Could you check a few things on this model? Use its own coordinates, in mm. Face numbers are marked on the shaded views. A direction names the side the tool comes from. Round coordinates to 2 decimals unless told otherwise and drop trailing zeros. Loops run counter-clockwise (first coordinate to the right, second up) from the corner with the lowest first, then second, coordinate; pieces in that order, holes last. Notation, with made-up numbers: M -31,54 L 23,54 A20 ccw 23,89 Z; hole C -33.75,9 d7. An arc over 180 degrees is marked long. Answer in a Markdown table with one row per item.
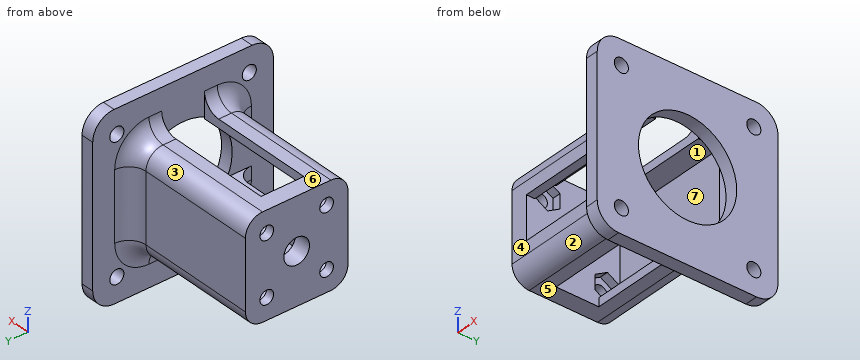
```python
from build123d import *

# Parameters (mm, degrees)
F0_W     = 24
F0_H     = 24
F0_R     = 1.6
F0_R_2   = 3
F1_DEPTH = 4
F4_DEPTH = 2
F5_DEPTH = 28
F6_W     = 42.3
F6_H     = 42.3
F6_R     = 1.65
F6_R_2   = 11.5
F7_DEPTH = 3
F8_R     = 5
F9_F1_R  = 4
F9_F2_R  = 4


with BuildPart() as f1:
    # F0 (on Right) → F1 (new body)
    with BuildSketch(Plane.YZ):
        Rectangle(F0_W, F0_H)
        with Locations((-7, -7)):
            Circle(F0_R, mode=Mode.SUBTRACT)
        with Locations((7, -7)):
            Circle(F0_R, mode=Mode.SUBTRACT)
        with Locations((-7, 7)):
            Circle(F0_R, mode=Mode.SUBTRACT)
        Circle(F0_R_2, mode=Mode.SUBTRACT)
        with Locations((7, 7)):
            Circle(F0_R, mode=Mode.SUBTRACT)
    extrude(amount=F1_DEPTH)

    # F2 (on face) → F4 (cut)
    with BuildSketch(Plane.YZ.offset(4)):
        Polygon((7, -3.6513684387), (4.1, -5.3256842194), (4.1, -8.6743157806), (7, -10.3486315613), (9.9, -8.6743157806), (9.9, -5.3256842194), align=None)
        Polygon((4.1, 5.3256842194), (7, 3.6513684387), (9.9, 5.3256842194), (9.9, 8.6743157806), (7, 10.3486315613), (4.1, 8.6743157806), align=None)
        Polygon((-9.9, 5.3256842194), (-7, 3.6513684387), (-4.1, 5.3256842194), (-4.1, 8.6743157806), (-7, 10.3486315613), (-9.9, 8.6743157806), align=None)
        Polygon((-4.1, -5.3256842194), (-7, -3.6513684387), (-9.9, -5.3256842194), (-9.9, -8.6743157806), (-7, -10.3486315613), (-4.1, -8.6743157806), align=None)
    extrude(amount=-F4_DEPTH, mode=Mode.SUBTRACT)

    # F3 (on face) → F5 (join)
    with BuildSketch(Plane.YZ.offset(4)):
        Polygon((-5, 12), (-12, 12), (-12, 5), (-10, 5), (-10, 10), (-5, 10), align=None)
        Polygon((12, 12), (5, 12), (5, 10), (10, 10), (10, -10), (5, -10), (5, -12), (12, -12), align=None)
        Polygon((-10, -5), (-12, -5), (-12, -12), (-5, -12), (-5, -10), (-10, -10), align=None)
    extrude(amount=F5_DEPTH)

    # F6 (on face) → F7 (join)
    with BuildSketch(Plane.YZ.offset(32)):
        Rectangle(F6_W, F6_H)
        with Locations((-15.5, -15.5)):
            Circle(F6_R, mode=Mode.SUBTRACT)
        with Locations((15.5, -15.5)):
            Circle(F6_R, mode=Mode.SUBTRACT)
        with Locations((-15.5, 15.5)):
            Circle(F6_R, mode=Mode.SUBTRACT)
        Circle(F6_R_2, mode=Mode.SUBTRACT)
        with Locations((15.5, 15.5)):
            Circle(F6_R, mode=Mode.SUBTRACT)
    extrude(amount=F7_DEPTH)

    # F8
    f8_edges = [f1.edges().sort_by_distance(p)[0] for p in [
        (33.5, 21.15, 21.15),
        (33.5, 21.15, -21.15),
        (33.5, -21.15, -21.15),
        (33.5, -21.15, 21.15),
    ]]
    fillet(f8_edges, radius=F8_R)

    # F9: fillet of radius 4 on 7 edges, made by hand

    # F9_f1
    f9_f1_edges = [f1.edges().sort_by_distance(p)[0] for p in [
        (16, 12, 12),
        (16, 12, -12),
        (16, -12, -12),
        (16, -12, 12),
    ]]
    fillet(f9_f1_edges, radius=F9_F1_R)

    # F9_f2
    f9_f2_edges = [f1.edges().sort_by_distance(p)[0] for p in [
        (32, 12, 0),
        (32, -6.5, -12),
        (32, -12, 6.5),
        (32, -10.8284271247, 10.8284271247),
        (32, -10.8284271247, -10.8284271247),
        (32, 10.8284271247, -10.8284271247),
        (32, 10.8284271247, 10.8284271247),
    ]]
    fillet(f9_f2_edges, radius=F9_F2_R)


solid = f1.part
```
1) I want a section at A-A, the plane z = 0. Please give me the cut outline in (x, y).
Computed:
| item | result |
|---|---|
| outline | M 0,-12 L 4,-12 L 4,-3 L 0,-3 Z; M 0,3 L 4,3 L 4,10 L 32,10 L 32,11.5 L 35,11.5 L 35,21.15 L 32,21.15 L 32,16 A4 cw 28,12 L 0,12 Z; M 32,-21.15 L 35,-21.15 L 35,-11.5 L 32,-11.5 Z |
2) If we mould it in two halves opening along Z, with no side actions, what happens to the marked faces 1, 2 and 3? For each: released by +Z, released by -Z, zero draft, split by the parting line, or undercut.
Computed:
| item | result |
|---|---|
| face 1 | undercut |
| face 2 | released by -Z |
| face 3 | released by +Z |
3) Will these pins go through, and if not, where does the flat tip stop? P1, Ø1.8, axis at x = 17.5, y = -11.5, coming from the -Z side; P2, Ø5, axis at x = 12, z = -14, coming from the -Y side; P3, Ø1.5, axis at x = 5, z = 10.5, coming from the +Y side.
Computed:
| item | result |
|---|---|
| P1 | stops at z = -11.04 |
| P2 | stops at y = -9.94 |
| P3 | stops at y = 11.6 |
4) I need wall thicknesses on line 1 (Z direction, x = 32.7, y = 15.5); line 2 (Y direction, x = 1, z = -7); line 3 (Z direction, x = 6.5, y = -8). Which ranges of each line are inside material? Lowest first, please.
Computed:
| item | result |
|---|---|
| line 1 | z = -21.15 to -17.15, -13.85 to 13.85, 17.15 to 21.15 |
| line 2 | y = -12 to -8.6, -5.4 to 5.4, 8.6 to 12 |
| line 3 | z = -12 to -10, 10 to 12 |
5) I want a section at C-C, the plane y = 1.5. Please give me the cut outline in (x, z).
Computed:
| item | result |
|---|---|
| outline | M 0,-12 L 4,-12 L 4,-2.6 L 0,-2.6 Z; M 0,2.6 L 4,2.6 L 4,12 L 0,12 Z; M 32,-21.15 L 35,-21.15 L 35,-11.4 L 32,-11.4 Z; M 32,11.4 L 35,11.4 L 35,21.15 L 32,21.15 Z |
6) Which directions (+Z, -Z, +X, -X, +Y, -Y) give clear straight access to the entire face, cutting with the end or side of a thin tool? Please do the marked faces 4, 5, 6 and 7.
Computed:
| item | result |
|---|---|
| face 4 | +Z, -Z, -X, -Y |
| face 5 | -Z, -X, +Y, -Y |
| face 6 | +Z, -X, +Y, -Y |
| face 7 | none |
7) I want a section at D-D, the plane z = 7. State how many separate pieces and enclosed holes the cut face has, plus the area to 3 significant figures.
Computed:
| item | result |
|---|---|
| separate pieces | 3 |
| enclosed holes | 0 |
| area | 251 mm² |
8) I want a section at B-B, the plane x = 7.5. Please give me the cut outline in (y, z).
Computed:
| item | result |
|---|---|
| outline | M -12,-8 A4 ccw -8,-12 L -5,-12 L -5,-10 L -10,-10 L -10,-5 L -12,-5 Z; M -12,5 L -10,5 L -10,10 L -5,10 L -5,12 L -8,12 A4 ccw -12,8 Z; M 5,-12 L 8,-12 A4 ccw 12,-8 L 12,8 A4 ccw 8,12 L 5,12 L 5,10 L 10,10 L 10,-10 L 5,-10 Z |
